Autodesk Inventor part; units mm, degrees
ref_plane "YZ Plane" through (0, 0, 0) normal (1, 0, 0) x (0, 1, 0)
ref_plane "XZ Plane" through (0, 0, 0) normal (0, 1, 0) x (-1, 0, 0)
ref_plane "XY Plane" through (0, 0, 0) normal (0, 0, 1) x (1, 0, 0)
sketch "Skizze1" plane through (0, 0, 0) normal (1, 0, 0) x (0, 1, 0)
  line L0 (384.3381, -178.6102) -> (384.3381, -313.6102)
  line L1 (384.3381, -313.6102) -> (584.3932, -631.3447)
  line L2 (584.3932, -631.3447) -> (669.3932, -631.3447)
  line L3 (669.3932, -631.3447) -> (384.3381, -178.6102)
  point P0 (0, 0)
  dimension "d0" = 135
  dimension "d1" = 85
  dimension "d2" = 535
  dimension "d3" = 375.4694
extrude "Extrusion1" add sketch "Skizze1" along normal blind 20
fillet "Rundung1" radius 2 4 edges at (20, 526.8656, -404.9774) (0, 526.8656, -404.9774) (20, 484.3656, -472.4774) (0, 484.3656, -472.4774)
properties part number "VerstaerkungHintenSchraeg"
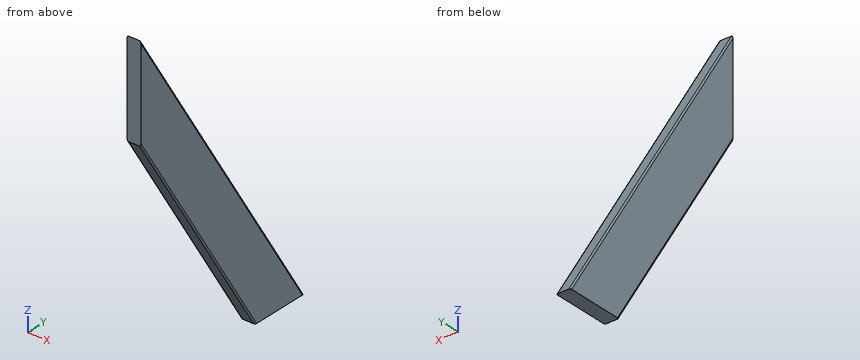
Model file for the job. Use its own axes, mm. Coordinates: 2 decimals unless noted, no trailing zeros. Loops run counter-clockwise (first coordinate to the right, second up) from the corner with the lowest first, then second, coordinate; pieces in that order, holes last. Notation, with made-up numbers: (24, 32.25) - (35, 32.25) arc R13 ccw to (35, 52.25) - close; hole circle Ø4 at (88, 59.5). An arc over 180 degrees is marked (long way). Answer as a JSON object with one key per item and string values. Group by question number.
(1) Probe line 1 along Y through (x, z) = (9.75, -524.5); line 2 along Z through (x, y) = (16.5, 551); line 3 along Z through (x, y) = (15.25, 526). List the from-to ranges inside material, lowest first.
(2) Flat gauge pins, fed straight in: pin 1 (1.5 mm diameter, centred on x = 12, z = -468.5, fed in from -Y); pin 2 (10 mm diameter, centred on x = 2.5, z = -300.5, fed in from +Y); pin 3 (4 mm diameter, centred on x = 10, y = 536.5, fed in from -Z); pin 4 (5 mm diameter, centred on y = 462, z = -313.5, fed in from -X). Where does each tip first touch, or does it go through?
(3) Cut at A-A (x = 12). Give the cut face in (y, z).
Geometry says:
{
 "1": {"line 1": "y = 517.12 to 602.12", "line 2": "z = -578.31 to -443.31", "line 3": "z = -538.6 to -403.6"},
 "2": {"pin 1": "stops at y = 481.39", "pin 2": "stops at y = 464.23", "pin 3": "stops at z = -558.46", "pin 4": "stops at x = 0"},
 "3": {"outline": "(384.34, -313.61) - (584.39, -631.34) - (669.39, -631.34) - (384.34, -178.61) - close"}
}
